Answer from the drawing. Dimensions are ordinates in mm from the lowest x, y and z of the part. Coordinates: 2 decimals unless noted, no trailing zeros. Write each loop counter-clockwise with the first axis right and the second up, starting at its lowest first coordinate (ties: lowest second). Pieces come first, ordered by that corner, then holes.
1) This flat-tipped pin is pushed along its axis until it touches: pin 1 Ø3 at (y, z) = (2, 17) entering from +X (1 decimal). Where does it stop, or does it pass through?
2) The part is cut by section D-D (x = 41.5). Determine the outline of the cut face in (y, z), then the cut area to 3 significant figures.
3) Determine the mould class of the marked faces 1, 2 and 3 for opening direction Z: +Z half, -Z half, draft (parallel to the pull), parting line (faces both ways), or undercut.
4) The part is cut by section A-A (x = 25.5). Determine the outline of the cut face in (y, z).
5) Find the intervals of material crossed by line 1 (Z direction, x = 16, y = 2.5); line 2 (X direction, y = 5.5, z = 29.5); line 3 (X direction, y = 1.25, z = 36) (1 decimal), in increasing order.
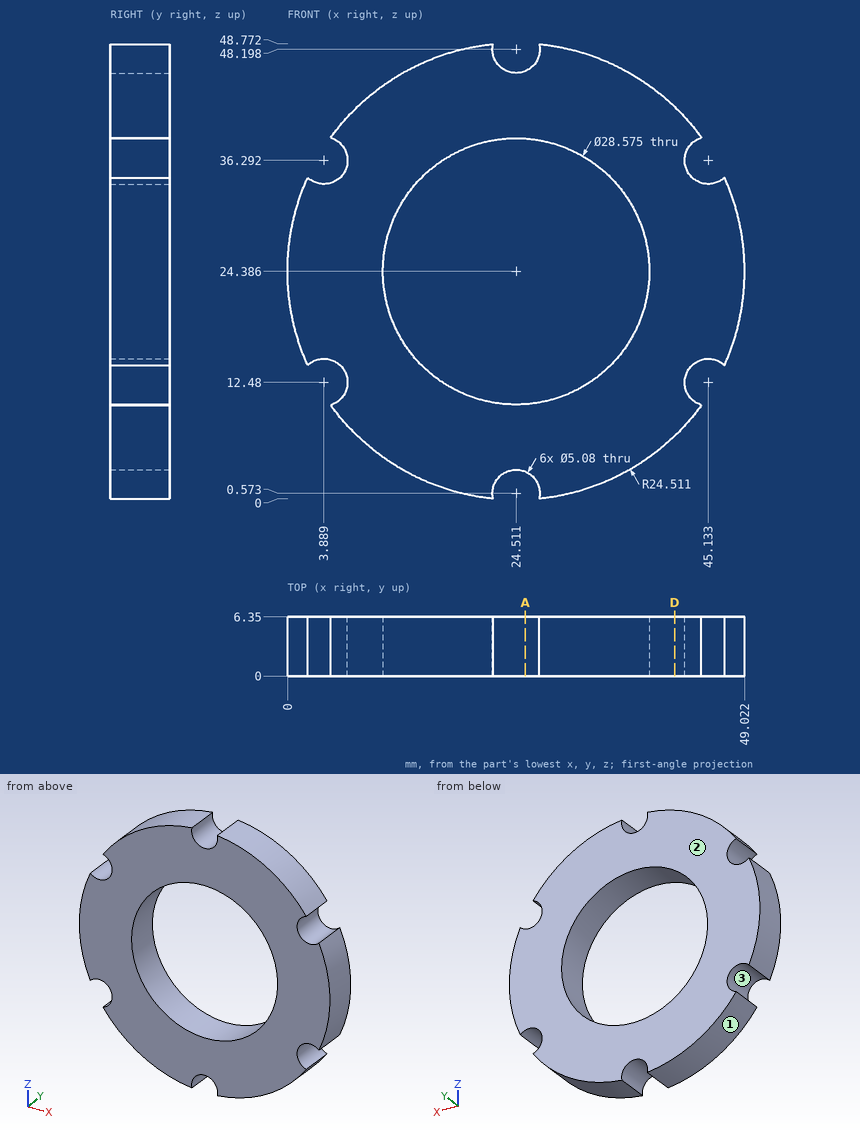
Reported:
1. pin 1: stops at x = 48.3
2. outline: (0, 6.72) - (6.35, 6.72) - (6.35, 42.05) - (0, 42.05) - close
2. area: 224 mm2
3. face 1: -Z half
3. face 2: draft
3. face 3: undercut
4. outline: (0, 2.91) - (6.35, 2.91) - (6.35, 10.13) - (0, 10.13) - close; (0, 38.64) - (6.35, 38.64) - (6.35, 45.86) - (0, 45.86) - close
5. line 1: z = 1.4 to 12.91, 35.86 to 47.37
5. line 2: x = 0.54 to 11.17, 37.85 to 48.48
5. line 3: x = 6.4 to 16.2, 32.8 to 42.6
